Geometry check sheet. Reference: the model listing, model coordinates, mm. Face numbers are marked on the shaded views. A direction names the side the tool comes from. Give positions to 0.01 mm unless a question says otherwise; leave off trailing zeros. Loops run counter-clockwise (first coordinate to the right, second up) from the corner with the lowest first, then second, coordinate; pieces in that order, holes last. Notation, with made-up numbers: (-30, -17.75) -> (-18, -17.75) arc R29 ccw to (-18, 21.25) -> close; hole circle Ø6 at (35.25, -21.5). An arc over 180 degrees is marked (long way). Answer as a JSON object with one key per item and string values.
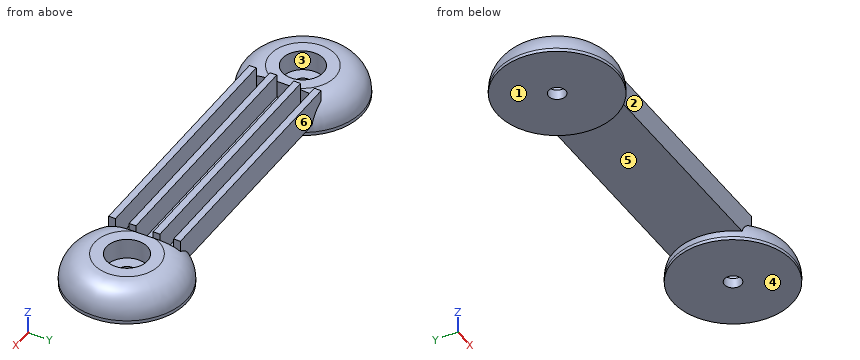
from build123d import *

# Parameters (mm, degrees)
CROQUIS1_R                = 17.5
SALIENTE_EXTRUIR1_DEPTH   = 9
SALIENTE_EXTRUIR1_2_DEPTH = 9
REDONDEO1_R               = 8
REDONDEO2_R               = 8
CROQUIS5_W                = 72
CROQUIS5_H                = 21
SALIENTE_EXTRUIR2_DEPTH   = 8
CROQUIS6_W                = 72
CROQUIS6_H                = 4
CROQUIS6_H_2              = 5
CORTAR_EXTRUIR1_DEPTH     = 7
CROQUIS8_R                = 6
CORTAR_EXTRUIR2_DEPTH     = 6
CROQUIS9_R                = 2.5
CORTAR_EXTRUIR3_DEPTH     = 66.394954068


with BuildPart() as part:
    # Croquis1 → Saliente-Extruir1 (new body)
    with BuildSketch(Plane.XY):
        with Locations((45, 0)):
            Circle(CROQUIS1_R)
    extrude(amount=SALIENTE_EXTRUIR1_DEPTH)

    # Redondeo2
    redondeo2_edges = [part.edges().sort_by_distance(p)[0] for p in [
        (27.5, 0, 9),
    ]]
    fillet(redondeo2_edges, radius=REDONDEO2_R)



with BuildPart() as body_2:
    # Croquis1 → Saliente-Extruir1 2 (new body)
    with BuildSketch(Plane.XY):
        with Locations((-45, 0)):
            Circle(CROQUIS1_R)
    extrude(amount=SALIENTE_EXTRUIR1_2_DEPTH)

    # Redondeo1
    redondeo1_edges = [body_2.edges().sort_by_distance(p)[0] for p in [
        (-62.5, 0, 9),
    ]]
    fillet(redondeo1_edges, radius=REDONDEO1_R)


with BuildPart() as part_1:
    add(part.part)

    add(body_2.part)  # Saliente-Extruir2 merges body 2
    # Croquis5 → Saliente-Extruir2 (add)
    with BuildSketch(Plane.XY.offset(3)):
        Rectangle(CROQUIS5_W, CROQUIS5_H)
    extrude(amount=SALIENTE_EXTRUIR2_DEPTH)

    # Croquis6 → Cortar-Extruir1 (cut)
    with BuildSketch(Plane.XY.offset(11)):
        with Locations((0, 6.5)):
            Rectangle(CROQUIS6_W, CROQUIS6_H)
        Rectangle(CROQUIS6_W, CROQUIS6_H_2)
        with Locations((0, -6.5)):
            Rectangle(CROQUIS6_W, CROQUIS6_H)
    extrude(amount=-CORTAR_EXTRUIR1_DEPTH, mode=Mode.SUBTRACT)

    # Croquis8 → Cortar-Extruir2 (cut)
    with BuildSketch(Plane.XY.offset(9)):
        with Locations((-45, 0)):
            Circle(CROQUIS8_R)
        with Locations((45, 0)):
            Circle(CROQUIS8_R)
    extrude(amount=-CORTAR_EXTRUIR2_DEPTH, mode=Mode.SUBTRACT)

    # Croquis9 → Cortar-Extruir3 (cut, through all)
    with BuildSketch(Plane.XY.offset(3)):
        with Locations((45, 0)):
            Circle(CROQUIS9_R)
        with Locations((-45, 0)):
            Circle(CROQUIS9_R)
    extrude(amount=-CORTAR_EXTRUIR3_DEPTH, mode=Mode.SUBTRACT)


solid = part_1.part
1) Draft check along X on the marked faces 4, 5 and 6. Enter one of: pulls with the +X half, pulls with the -X half, needs draft (parallel to the pull), parting line crosses it, or undercut.
Geometry check:
{"face 4": "needs draft", "face 5": "undercut", "face 6": "undercut"}
2) Tool access check on the marked faces 1, 2 and 3. Record the directions out of +Z, -Z, +X, -X, +Y, -Y that give a thin tool (end or side, any length) a straight path to the whole face; none if there is none.
Geometry check:
{"face 1": "-Z, +X, -X, +Y, -Y", "face 2": "+Z, -Y", "face 3": "+Z"}
3) Depth check by flat-ended pin: P1, Ø2.5, axis at y = 0.5, z = 7, coming from the -X side; P2, Ø9, axis at x = -43, y = 2.5, coming from the +Z side; P3, Ø0.6, axis at y = -3, z = 10.5, coming from the -X side. Enter the tip coordinate at first touch or a pass-through.
Geometry check:
{"P1": "stops at x = -60.93", "P2": "stops at z = 9", "P3": "stops at x = -36"}
4) Section check C-C on x = 9. Record the cut outline in (y, z), plus the area to 3 significant figures.
Geometry check:
{"outline": "(-10.5, 3) -> (10.5, 3) -> (10.5, 11) -> (8.5, 11) -> (8.5, 4) -> (4.5, 4) -> (4.5, 11) -> (2.5, 11) -> (2.5, 4) -> (-2.5, 4) -> (-2.5, 11) -> (-4.5, 11) -> (-4.5, 4) -> (-8.5, 4) -> (-8.5, 11) -> (-10.5, 11) -> close", "area": "77.0 mm2"}
5) Section check A-A on x = -45. Record the cut outline in (y, z).
Geometry check:
{"outline": "(-17.5, 0) -> (-2.5, 0) -> (-2.5, 3) -> (-6, 3) -> (-6, 9) -> (-9.5, 9) arc R8 ccw to (-17.5, 1) -> close; (2.5, 0) -> (17.5, 0) -> (17.5, 1) arc R8 ccw to (9.5, 9) -> (6, 9) -> (6, 3) -> (2.5, 3) -> close"}
6) Section check B-B on y = 0. Count the separate pieces of the cut face and the enclosed holes in it, plus the area to 3 significant figures.
Geometry check:
{"separate pieces": "3", "enclosed holes": "0", "area": "398 mm2"}
7) Material ranges on line 1 along Y through (x, z) = (7.5, 6); line 2 along Y through (x, z) = (-45, 1.3); line 3 along X through (y, z) = (0.5, 6.25), recorded low to high. Write a range as from..to.
Geometry check:
{"line 1": "y = -10.5..-8.5, -4.5..-2.5, 2.5..4.5, 8.5..10.5", "line 2": "y = -17.49..-2.5, 2.5..17.49", "line 3": "x = -60.53..-50.98, -39.02..-36, 36..39.02, 50.98..60.53"}
